Design review of the part shown in the three views and the two pictorial views. Dimensions are in mm from the part's minimum x, y and z. Round coordinates to 2 decimals unless told otherwise and drop trailing zeros. Loops run counter-clockwise (first coordinate to the right, second up) from the corner with the lowest first, then second, coordinate; pieces in that order, holes last. Notation, with made-up numbers: M 44,17 L 103,17 A26 cw 103,33 Z; hole C -36,57 d10. An arc over 180 degrees is marked long. Answer as CSV lines item,"result". Start each with the question number.
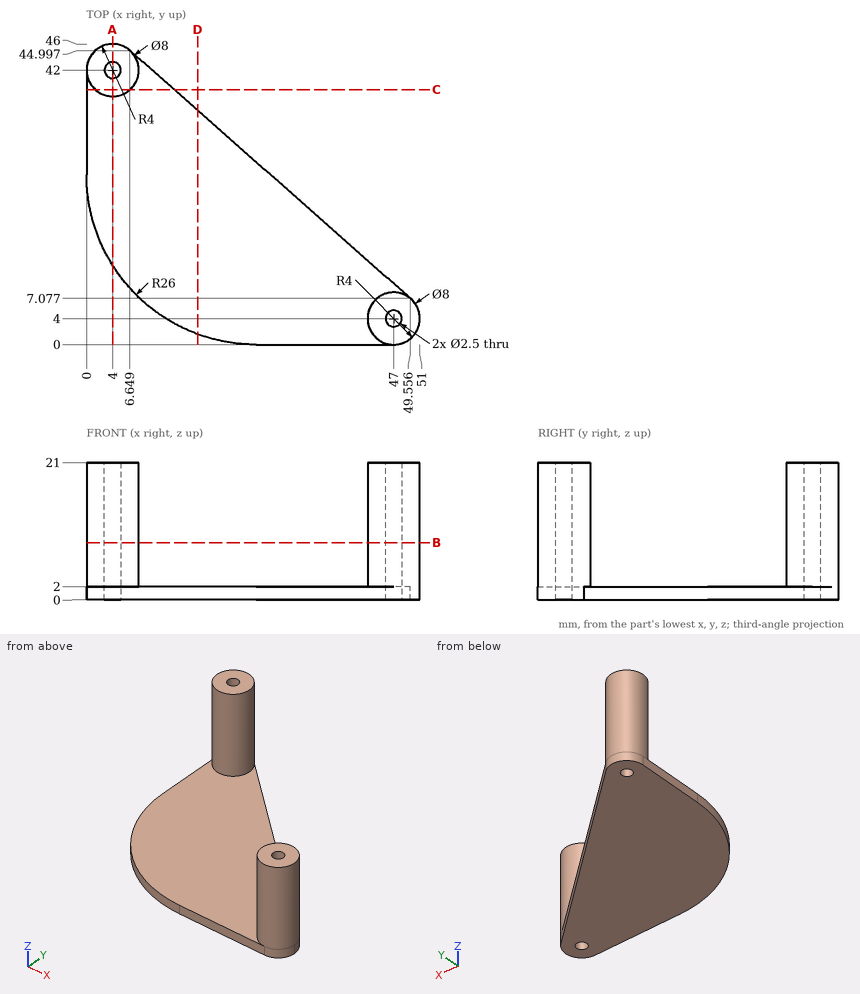
Item 1: Consider section A-A, the plane x = 4. Write out the cut boundary in (y, z), then the cut area to 3 significant figures.
Item 2: Consider section B-B, the plane z = 8.75. Write out the cut boundary in (x, y), then the cut area to 3 significant figures.
Item 3: Consider section D-D, the plane x = 17. Write out the cut boundary in (y, z).
Item 4: To check wall thickness, follow line 1 (Y direction, x = 47, z = 13.75); line 2 (Y direction, x = 4, z = 12); line 3 (Z direction, x = 35, y = 11). State the ranges of each line that lie inside material, in increasing order.
Item 5: Consider section C-C, the plane y = 39. Write out the cut boundary in (x, z) (1 decimal), then the cut area to 3 significant figures.
Item 6: Insertion check: pin 1 Ø3 at (x, y) = (4, 42) entering from -Z; pin 2 Ø12 at (x, y) = (8.5, 14) entering from +Z. Each pin has a flat end and moves straight along its axis. Give the tip position at first contact, or say it passes through.
Found:
1,outline,"M 12.14,0 L 40.75,0 L 40.75,21 L 38,21 L 38,2 L 12.14,2 Z; M 43.25,0 L 46,0 L 46,21 L 43.25,21 Z"
1,area,"167 mm^2"
2,outline,"C 4,42 d8; C 47,4 d8; hole C 4,42 d2.5; hole C 47,4 d2.5"
2,area,"90.7 mm^2"
3,outline,"M 1.61,0 L 35.85,0 L 35.85,2 L 1.61,2 Z"
4,line 1,"y = 0 to 2.75, 5.25 to 8"
4,line 2,"y = 38 to 40.75, 43.25 to 46"
4,line 3,"z = 0 to 2"
5,outline,"M 0,0 L 13.4,0 L 13.4,2 L 6.6,2 L 6.6,21 L 1.4,21 L 1.4,2 L 0,2 Z"
5,area,"127 mm^2"
6,pin 1,"stops at z = 0"
6,pin 2,"stops at z = 2"
